```python
from build123d import *

# Parameters (mm, degrees)
SKETCH1_W                   = 50.8
SKETCH1_H                   = 50.8
BOSS_EXTRUDE1_DEPTH         = 12.7
SKETCH2_W                   = 25.4
SKETCH2_H                   = 25.4
CUT_EXTRUDE1_DEPTH          = 26.4
SKETCH3_W                   = 25.4
SKETCH3_H                   = 25.4
SKETCH3_W_2                 = 22.1742
SKETCH3_H_2                 = 22.1742
CUT_EXTRUDE2_DEPTH          = 22.86
SKETCH5_W                   = 25.4
SKETCH5_H                   = 25.4
SKETCH5_W_2                 = 22.1742
SKETCH5_H_2                 = 22.1742
CUT_EXTRUDE4_DEPTH          = 22.86
SKETCH7_R                   = 3.3
CUT_EXTRUDE6_DEPTH          = 26.4
TAP_DRILL_FOR_M6X1_0_TAP1_D = 5


with BuildPart() as part:
    # Sketch1 → Boss-Extrude1 (new body, symmetric)
    with BuildSketch(Plane.XY):
        Rectangle(SKETCH1_W, SKETCH1_H)
    extrude(amount=BOSS_EXTRUDE1_DEPTH, both=True)

    # Sketch2 → Cut-Extrude1 (cut, through all)
    with BuildSketch(Plane.XY.offset(12.7)):
        with Locations((12.7, 12.7)):
            Rectangle(SKETCH2_W, SKETCH2_H)
    extrude(amount=-CUT_EXTRUDE1_DEPTH, mode=Mode.SUBTRACT)

    # Sketch3 → Cut-Extrude2 (cut)
    with BuildSketch(Plane(origin=(25.4, 0, 0), x_dir=(0, 0, -1), z_dir=(1, 0, 0))):
        with Locations((0, -12.7)):
            Rectangle(SKETCH3_W, SKETCH3_H)
        with Locations((0, -12.7)):
            Rectangle(SKETCH3_W_2, SKETCH3_H_2, mode=Mode.SUBTRACT)
    extrude(amount=-CUT_EXTRUDE2_DEPTH, mode=Mode.SUBTRACT)

    # Sketch5 → Cut-Extrude4 (cut)
    with BuildSketch(Plane(origin=(0, 25.4, 0), x_dir=(1, 0, 0), z_dir=(0, 1, 0))):
        with Locations((-12.7, 0)):
            Rectangle(SKETCH5_W, SKETCH5_H)
        with Locations((-12.7, 0)):
            Rectangle(SKETCH5_W_2, SKETCH5_H_2, mode=Mode.SUBTRACT)
    extrude(amount=-CUT_EXTRUDE4_DEPTH, mode=Mode.SUBTRACT)

    # Sketch7 → Cut-Extrude6 (cut, through all)
    with BuildSketch(Plane.XY.offset(12.7)):
        with Locations((-12.7, -12.7)):
            Circle(SKETCH7_R)
    extrude(amount=-CUT_EXTRUDE6_DEPTH, mode=Mode.SUBTRACT)

    # Tap Drill for M6x1.0 Tap1 (through all)
    with Locations(Plane.XY.offset(11.0871)):
        with Locations((14.54, -12.6979), (-12.6979, 14.54)):
            Hole(TAP_DRILL_FOR_M6X1_0_TAP1_D / 2)


solid = part.part
```
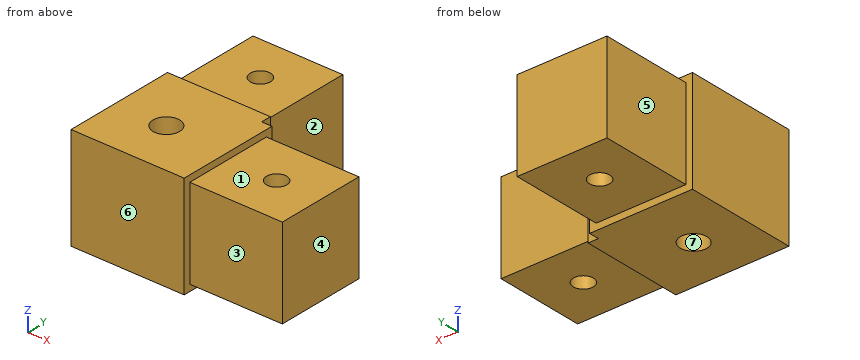
For this review, take the finished solid that the model builds, in its own axes (mm). Face numbers are marked on the shaded views. A direction names the side the tool comes from. Coordinates: 2 decimals unless noted, no trailing zeros. Write each loop counter-clockwise with the first axis right and the second up, starting at its lowest first coordinate (ties: lowest second). Pieces come first, ordered by that corner, then holes. Notation, with made-up numbers: (45.25, 88.25) - (53.25, 88.25) arc R16 cw to (53.25, 95.25) - close; hole circle Ø4 at (63.5, -19.75). An arc over 180 degrees is marked (long way). Answer in a Markdown table with one row per item. Add a question column.
Q1. We need section D-D, the plane y = -22. State the section outline as (x, z) points.
Q2. Draft analysis for pull direction X (two halves, no side actions). For the marked faces 4, 5, 6 and 7, state which applies: +X half, -X half, draft (parallel to the pull), parting line (faces both ways), or undercut.
Q3. We need section B-B, the plane x = -12.7. State the section outline as (y, z) points, and give its area (3 significant figures).
Q4. We need section C-C, the plane z = 2. State the section outline as (x, y) points, and give its area (3 significant figures).
Q5. For P1, Ø6.5, axis at x = -17, y = 11.5, coming from the +Z side; P2, Ø12, axis at x = 4, y = 9.5, coming from the -Z side; P3, Ø11, axis at y = 12, z = -5.5, coming from the -X side; P4, Ø1.5, axis at x = 15.5, y = 0, coming from the +Z side, all flat-tipped, find the tip position at first contact; note any pin that passes through.
Q6. Tool access review of the marked faces 1, 2 and 3: name each direction out of +Z, -Z, +X, -X, +Y, -Y from which nothing blocks a thin tool from reaching the whole face with its end or side.
Q7. We need section A-A, the plane x = 14.54. State the section outline as (y, z) points.
Q8. For probe 1 along Y at (x, z) = (-12.7, -0.5); probe 2 along Y at (x, z) = (-13, 7); probe 3 along Y at (x, z) = (14.54, 5.25), list the stretches that pass through material, from the lowest coordinate up.
Answer list:
| question | item | result |
|---|---|---|
| 1 | outline | (-25.4, -12.7) - (2.54, -12.7) - (2.54, -11.09) - (25.4, -11.09) - (25.4, 11.09) - (2.54, 11.09) - (2.54, 12.7) - (-25.4, 12.7) - close |
| 2 | face 4 | +X half |
| 2 | face 5 | -X half |
| 2 | face 6 | draft |
| 2 | face 7 | undercut |
| 3 | outline | (-25.4, -12.7) - (-16, -12.7) - (-16, 12.7) - (-25.4, 12.7) - close; (-9.4, -12.7) - (2.54, -12.7) - (2.54, -11.09) - (12.04, -11.09) - (12.04, 11.09) - (2.54, 11.09) - (2.54, 12.7) - (-9.4, 12.7) - close; (17.04, -11.09) - (25.4, -11.09) - (25.4, 11.09) - (17.04, 11.09) - close |
| 3 | area | 938 mm2 |
| 4 | outline | (-25.4, -25.4) - (2.54, -25.4) - (2.54, -23.79) - (25.4, -23.79) - (25.4, -1.61) - (2.54, -1.61) - (2.54, 0) - (0, 0) - (0, 2.54) - (-1.61, 2.54) - (-1.61, 25.4) - (-23.79, 25.4) - (-23.79, 2.54) - (-25.4, 2.54) - close; hole circle Ø6.6 at (-12.7, -12.7); hole circle Ø5 at (-12.7, 14.54); hole circle Ø5 at (14.54, -12.7) |
| 4 | area | 1,710 mm2 |
| 5 | P1 | stops at z = 11.09 |
| 5 | P2 | stops at z = -11.09 |
| 5 | P3 | stops at x = -23.79 |
| 5 | P4 | passes through |
| 6 | face 1 | +Z, +X, +Y, -Y |
| 6 | face 2 | +Z, -Z, +X, +Y |
| 6 | face 3 | +Z, -Z, +X, -Y |
| 7 | outline | (-23.79, -11.09) - (-15.2, -11.09) - (-15.2, 11.09) - (-23.79, 11.09) - close; (-10.2, -11.09) - (-1.61, -11.09) - (-1.61, 11.09) - (-10.2, 11.09) - close |
| 8 | probe 1 | y = -25.4 to -16, -9.4 to 12.04, 17.04 to 25.4 |
| 8 | probe 2 | y = -25.4 to -15.99, -9.41 to 12.06, 17.02 to 25.4 |
| 8 | probe 3 | y = -23.79 to -15.2, -10.2 to -1.61 |
